from build123d import *

# Parameters (mm, degrees)
SKETCH1_W           = 34
SKETCH1_H           = 42
BOSS_EXTRUDE1_DEPTH = 37
CUT_EXTRUDE1_DEPTH  = 9
CUT_EXTRUDE2_DEPTH  = 9
SKETCH9_R           = 25
BOSS_EXTRUDE3_DEPTH = 42
SKETCH10_W          = 16
SKETCH10_H          = 34
CUT_EXTRUDE5_DEPTH  = 70.978568148
CUT_EXTRUDE6_DEPTH  = 5
SKETCH13_W          = 8
SKETCH13_H          = 26
CUT_EXTRUDE7_DEPTH  = 89.051121515


with BuildPart() as part:
    # Sketch1 → Boss-Extrude1 (new, symmetric)
    with BuildSketch(Plane.XY):
        with Locations((17, 21)):
            Rectangle(SKETCH1_W, SKETCH1_H)
    extrude(amount=BOSS_EXTRUDE1_DEPTH, both=True)

    # Sketch2 → Cut-Extrude1 (cut)
    with BuildSketch(Plane.XY.offset(37)):
        Polygon((17, 42), (9, 42), (9, 0), (17, 0), (25, 0), (25, 42), align=None)
    extrude(amount=-CUT_EXTRUDE1_DEPTH, mode=Mode.SUBTRACT)

    # Sketch3 → Cut-Extrude2 (cut)
    with BuildSketch(Plane(origin=(0, 0, -37), x_dir=(-1, 0, 0), z_dir=(0, 0, -1))):
        Polygon((-17, 42), (-25, 42), (-25, 0), (-17, 0), (-9, 0), (-9, 42), align=None)
    extrude(amount=-CUT_EXTRUDE2_DEPTH, mode=Mode.SUBTRACT)

    # Sketch9 → Boss-Extrude3 (add, through all)
    with BuildSketch(Plane(origin=(0, 0, 0), x_dir=(1, 0, 0), z_dir=(0, 1, 0))):
        with Locations((17, 0)):
            Circle(SKETCH9_R)
    extrude(amount=BOSS_EXTRUDE3_DEPTH)

    # Sketch10 → Cut-Extrude5 (cut, through all)
    with BuildSketch(Plane(origin=(0, 42, 0), x_dir=(1, 0, 0), z_dir=(0, 1, 0))):
        with Locations((16.53776174, 0)):
            Rectangle(SKETCH10_W, SKETCH10_H)
    extrude(amount=-CUT_EXTRUDE5_DEPTH, mode=Mode.SUBTRACT)

    # Sketch11 → Cut-Extrude6 (cut)
    with BuildSketch(Plane.ZY.offset(-24.53776174)):
        Polygon((0, 42), (-10, 42), (-10, 32), (10, 32), (10, 42), align=None)
    extrude(amount=-CUT_EXTRUDE6_DEPTH, mode=Mode.SUBTRACT)

    # Sketch13 → Cut-Extrude7 (cut, through all)
    with BuildSketch(Plane(origin=(0, 0, -28), x_dir=(-1, 0, 0), z_dir=(0, 0, -1))):
        with Locations((-17, 21)):
            Rectangle(SKETCH13_W, SKETCH13_H)
    extrude(amount=-CUT_EXTRUDE7_DEPTH, mode=Mode.SUBTRACT)


solid = part.part
Part model, mm, in its own coordinate system. A direction names the side the tool comes from. Give positions to 0.01 mm unless a question says otherwise; leave off trailing zeros. Loops run counter-clockwise (first coordinate to the right, second up) from the corner with the lowest first, then second, coordinate; pieces in that order, holes last.
(1) 3-axis set-ups, long thin cutter, end or side, ignore diameter. For faces 5 (the flat face through (29.538, 37, 0)), 6 (the flat face through (34, 21, -28)), 7 (the flat face through (17, 34, 22)): which of +Z, -Z, +X, -X, +Y, -Y reach the whole face in a straight line?
Return value:
face 5: +Y
face 6: -Z, +X, +Y, -Y
face 7: +Z, -Z
(2) Band-saw the part on B-B (y = 16). Write the cut outline in (x, z), and give its area (3 significant figures).
Return value:
outline: (0, -37) - (9, -37) - (9, -28) - (13, -28) - (13, -17) - (8.54, -17) - (8.54, 17) - (13, 17) - (13, 28) - (9, 28) - (9, 37) - (0, 37) - (0, 18.33) arc R25 ccw to (0, -18.33) - close; (21, -28) - (25, -28) - (25, -37) - (34, -37) - (34, -18.33) arc R25 ccw to (34, 18.33) - (34, 37) - (25, 37) - (25, 28) - (21, 28) - (21, 17) - (24.54, 17) - (24.54, -17) - (21, -17) - close
area: 1,910 mm2
(3) Drill centre lines: line 1 along Z through (x, y) = (27, 38); line 2 along X through (y, z) = (13.5, 30); line 3 along X through (y, z) = (31, -22.5). Where is each one in solid material? Low to high.
Return value:
line 1: z = -37 to -10, 10 to 37
line 2: x = 0 to 9, 25 to 34
line 3: x = 0 to 13, 21 to 34
(4) Pin check, flat tips, straight feed: pin 1 (20.5 mm diameter, centred on y = 18.5, z = 25, fed in from -X); pin 2 (9.5 mm diameter, centred on y = 24.5, z = -31, fed in from +X); pin 3 (4.5 mm diameter, centred on y = 12, z = -34, fed in from -X). Stop position of each tip, or through.
Return value:
pin 1: stops at x = -3.19
pin 2: stops at x = 34
pin 3: stops at x = 0
(5) Band-saw the part on A-A (x = 18). Write the cut outline in (y, z), and give its area (3 significant figures).
Return value:
outline: (0, -28) - (8, -28) - (8, -17) - (0, -17) - close; (0, 17) - (8, 17) - (8, 28) - (0, 28) - close; (34, -28) - (42, -28) - (42, -17) - (34, -17) - close; (34, 17) - (42, 17) - (42, 28) - (34, 28) - close
area: 352 mm2
(6) Pull direction Y, two halves, no side cores. Call faces 1 (the flat face through (27, 32, 0)), 2 (the flat face through (13, 21, 22)), 3 (the cylindrical face through (-8, 21, 0)), 4 (the flat face through (21, 21, 22)): pulls with the +Y half, pulls with the -Y half, needs draft (parallel to the pull), parting line crosses it, or undercut.
Return value:
face 1: pulls with the +Y half
face 2: undercut
face 3: needs draft
face 4: undercut
(7) Band-saw the part on C-C (z = -20.5). Write the cut outline in (x, y), and give its area (3 significant figures).
Return value:
outline: (0, 0) - (34, 0) - (34, 42) - (0, 42) - close; hole (13, 8) - (21, 8) - (21, 34) - (13, 34) - close
area: 1,220 mm2
(8) Band-saw the part on D-D (y = 7). Write the cut outline in (x, z), and give its area (3 significant figures).
Return value:
outline: (0, -37) - (9, -37) - (9, -28) - (25, -28) - (25, -37) - (34, -37) - (34, -18.33) arc R25 ccw to (34, 18.33) - (34, 37) - (25, 37) - (25, 28) - (9, 28) - (9, 37) - (0, 37) - (0, 18.33) arc R25 ccw to (0, -18.33) - close; hole (8.54, -17) - (24.54, -17) - (24.54, 17) - (8.54, 17) - close
area: 2,090 mm2
